from build123d import *

# Parameters (mm, degrees)
F1_DEPTH     = 34.29
F2_T1_DEPTH  = 46.9101181819
F2_T4_ANGLE  = 100.0995199097
F2_T6_ANGLE  = 150.1003280787
F2_T8_ANGLE  = 150.1003280787
F2_T10_ANGLE = 100.0995199097
F4_DEPTH     = 64.008
F5_SIZE      = 5.08


# Not quite as in the source:
# - a fillet or chamfer that OpenCascade refuses, or shapes differently, is made with other operations: its cross-section is extruded or revolved along the edge and cut away or added


with BuildPart() as f1:
    # F0 (on Front) → F1 (new body)
    with BuildSketch(Plane.XZ):
        with BuildLine():
            Line((23.1983069149, 22.5941853283), (-24.4065547209, 22.5941853283))
            Line((-24.4065547209, 22.5941853283), (-56.7875248861, 5.9204018954))
            ThreePointArc((-56.7875248861, 5.9204018954), (-58.6318372817, 3.0305487818), (-57.02917908, 0))
            Line((-57.02917908, 0), (-24.4065547209, -7.3702961741))
            Line((-24.4065547209, -7.3702961741), (23.1983069149, -7.3702961741))
            ThreePointArc((23.1983069149, -7.3702961741), (29.0260188517, -1.9620688543), (36.7306560898, 0))
            Line((36.7306560898, 0), (57.5124751139, 0))
            Line((57.5124751139, 0), (57.5124751139, 18.2445040364))
            Line((57.5124751139, 18.2445040364), (36.7306560898, 18.2445040364))
            ThreePointArc((36.7306560898, 18.2445040364), (29.6235434283, 19.3586478737), (23.1983069149, 22.5941853283))
        make_face()
    extrude(amount=F1_DEPTH)

    # F2: chamfer of 10.16 on 4 edges, made by hand

    # F2_s2 → F2_t1 (cut)
    with BuildSketch(Plane.YZ.offset(36.7306560898)):
        Polygon((-24.13, 18.2445040364), (-34.29, 8.0845040364), (-34.29, 18.2445040364), align=None)
        Polygon((-24.13, 0), (-34.29, 10.16), (-34.29, 0), align=None)
        Polygon((-10.16, 0), (0, 10.16), (0, 0), align=None)
        Polygon((-10.16, 18.2445040364), (0, 8.0845040364), (0, 18.2445040364), align=None)
    extrude(amount=F2_T1_DEPTH, mode=Mode.SUBTRACT)

    # F2_s3 → F2_t4 (revolve, cut)
    with BuildSketch(Plane.YZ.offset(36.7306560898)):
        Polygon((-10.16, 18.2445040364), (0, 8.0845040364), (0, 18.2445040364), align=None)
    revolve(axis=Axis((36.7306560898, 0, 41.469677098), (0, 1, 0)), revolution_arc=F2_T4_ANGLE, mode=Mode.SUBTRACT)

    # F2_s5 → F2_t6 (revolve, cut)
    with BuildSketch(Plane(origin=(34.5645844349, 0, -19.8752542161), x_dir=(0, 1, 0), z_dir=(0.8668996033, 0, -0.4984827758))):
        Polygon((-10.16, -11.7629612563), (0, -21.9229612563), (0, -11.7629612563), align=None)
    revolve(axis=Axis((36.7306560898, 0, -16.1082902421), (0, 1, 0)), revolution_arc=F2_T6_ANGLE, mode=Mode.SUBTRACT)

    # F2_s7 → F2_t8 (revolve, cut)
    with BuildSketch(Plane(origin=(34.5645844349, 0, -19.8752542161), x_dir=(0, 1, 0), z_dir=(0.8668996033, 0, -0.4984827758))):
        Polygon((-24.13, -11.7629612563), (-34.29, -21.9229612563), (-34.29, -11.7629612563), align=None)
    revolve(axis=Axis((36.7306560898, -34.29, -16.1082902421), (0, 1, 0)), revolution_arc=F2_T8_ANGLE, mode=Mode.SUBTRACT)

    # F2_s9 → F2_t10 (revolve, cut)
    with BuildSketch(Plane.YZ.offset(36.7306560898)):
        Polygon((-24.13, 18.2445040364), (-34.29, 8.0845040364), (-34.29, 18.2445040364), align=None)
    revolve(axis=Axis((36.7306560898, -34.29, 41.469677098), (0, 1, 0)), revolution_arc=F2_T10_ANGLE, mode=Mode.SUBTRACT)

    # F3 (on Top) → F4 (cut)
    with BuildSketch(Plane.XY):
        with BuildLine():
            Line((4.6636075713, -11.2218027934), (-10.7845906168, -11.2218027934))
            ThreePointArc((-10.7845906168, -11.2218027934), (-16.1768863909, -16.6140985675), (-10.7845906168, -22.0063943416))
            Line((-10.7845906168, -22.0063943416), (4.6636075713, -22.0063943416))
            ThreePointArc((4.6636075713, -22.0063943416), (10.0559033453, -16.6140985675), (4.6636075713, -11.2218027934))
        make_face()
    extrude(amount=F4_DEPTH, mode=Mode.SUBTRACT)

    # F5
    f5_edges = [f1.edges().sort_by_distance(p)[0] for p in [
        (57.512475, -28.691126, 13.683378),
        (57.512475, -17.145, 18.244504),
        (57.512475, -5.598874, 13.683378),
        (57.512475, -17.145, 0),
        (57.512475, -28.691126, 4.561126),
        (57.512475, -5.598874, 4.561126),
    ]]
    chamfer(f5_edges, length=F5_SIZE)


solid = f1.part
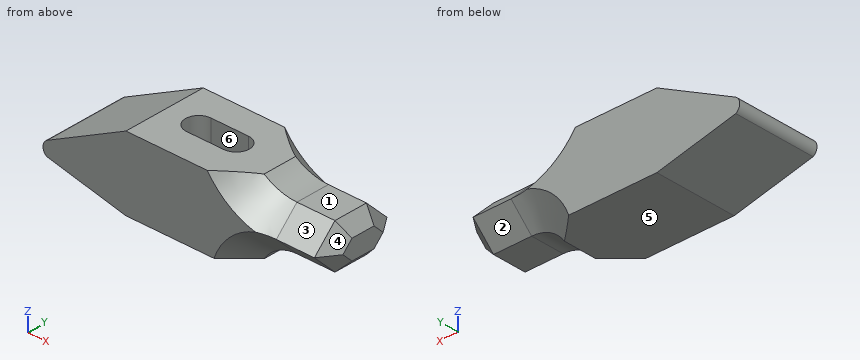
Build history of the part. All positions in model axes, mm. Face numbers are marked on the shaded views. A direction names the side the tool comes from. Coordinates: 2 decimals unless noted, no trailing zeros. Order: outer loops, then holes, each group sorted by start corner. A loop starts at its lowest first (then second) coordinate and runs counter-clockwise, first axis right, second up. Notation, with made-up numbers: (45.5, 70.25) -> (89.5, 70.25) arc R10 cw to (89.5, 80.25) -> close; hole circle Ø6 at (-21.5, 70.25). An arc over 180 degrees is marked (long way). One line per item, written item: value.
(1) Slice it at A-A, the plane y = -30. List the corners of the cut face in (x, z), plus the area to 3 significant figures.
Checked values:
outline: (-57.03, 0) -> (-24.41, -7.37) -> (16.56, -7.37) arc R21.98 cw to (36.73, 5.87) -> (52.43, 5.87) -> (54.73, 9.12) -> (52.43, 12.37) -> (36.73, 12.37) arc R29.1 cw to (14.59, 22.59) -> (-24.41, 22.59) -> (-56.79, 5.92) arc R3.41 ccw to start
area: 2,180 mm2
(2) Slice it at D-D, the plane y = -14. List the corners of the cut face in (x, z), plus the area to 3 significant figures.
Checked values:
outline: (-57.03, 0) -> (-24.41, -7.37) -> (23.2, -7.37) arc R16.11 cw to (36.73, 0) -> (52.43, 0) -> (57.51, 5.08) -> (57.51, 13.16) -> (52.43, 18.24) -> (36.73, 18.24) arc R23.23 cw to (23.2, 22.59) -> (9.38, 22.59) -> (9.38, 0) -> (-15.5, 0) -> (-15.5, 22.59) -> (-24.41, 22.59) -> (-56.79, 5.92) arc R3.41 ccw to start
area: 2,100 mm2
(3) Drop flat-ended pins along their axis: pin 1 Ø12.5 at (x, z) = (-2.5, 13.5) entering from +Y; pin 2 Ø4 at (x, y) = (41, -14.5) entering from -Z; pin 3 Ø5.5 at (x, y) = (-1, -17) entering from +Z; pin 4 Ø15.5 at (x, y) = (41, -17) entering from +Z. Give the stop position or say it passes through.
Checked values:
pin 1: y = 0
pin 2: z = 0
pin 3: z = 0
pin 4: z = 18.51
(4) Probe line 1 (Y direction, x = -2, z = 8.75); line 2 (Z direction, x = -7.5, y = -13.5); line 3 (X direction, y = -18, z = 13.25). List the from-to ranges inside material, lowest first. Write a range as [from, to].
Checked values:
line 1: [-34.29, -22.01], [-11.22, 0]
line 2: [-7.37, 0]
line 3: [-42.55, -16], [9.87, 57.43]
(5) Tool access for the marked faces 1, 2 and 3: list every direction of +Z, -Z, +X, -X, +Y, -Y with a clear straight run to the whole face (end or side of a thin tool).
Checked values:
face 1: +Z, +X, +Y, -Y
face 2: -Z, +X, +Y
face 3: +Z, +X, -Y
(6) Mould opens along X. For the marked faces 4, 5 and 6 say: pulls with the +X half, pulls with the -X half, needs draft (parallel to the pull), parting line crosses it, or undercut.
Checked values:
face 4: pulls with the +X half
face 5: needs draft
face 6: undercut
(7) Slice it at B-B, the plane x = -40.5. List the corners of the cut face in (y, z), plus the area to 3 significant figures.
Checked values:
outline: (-34.29, -3.73) -> (0, -3.73) -> (0, 14.31) -> (-34.29, 14.31) -> close
area: 619 mm2
(8) Slice it at C-C, the plane y = -7. List the corners of the cut face in (x, z), plus the area to 3 significant figures.
Checked values:
outline: (-57.03, 0) -> (-24.41, -7.37) -> (19.56, -7.37) arc R19.27 cw to (36.73, 3.16) -> (52.43, 3.16) -> (56.65, 9.12) -> (52.43, 15.08) -> (36.73, 15.08) arc R26.39 cw to (18.29, 22.59) -> (-24.41, 22.59) -> (-56.79, 5.92) arc R3.41 ccw to start
area: 2,410 mm2
